```python
from build123d import *

# Parameters (mm, degrees)
BOSS_EXTRU_1_DEPTH                                 = 50
CHAMBRAGE_POUR_VIS_T_TE_HEXAGONALE_M62_D           = 6.6
CHAMBRAGE_POUR_VIS_T_TE_HEXAGONALE_M62_CBORE_D     = 11
CHAMBRAGE_POUR_VIS_T_TE_HEXAGONALE_M62_CBORE_DEPTH = 6.4
ESQUISSE5_R                                        = 10
ENL_V_MAT_EXTRU_1_DEPTH                            = 64.472923802


with BuildPart() as part:
    # Esquisse1 → Boss.-Extru.1 (new body)
    with BuildSketch(Plane.XY):
        with BuildLine():
            Line((-36.108337762, -1), (-36.108337762, -16))
            Line((-36.108337762, -16), (13.891662238, -16))
            Line((13.891662238, -16), (13.891662238, -1))
            Line((13.891662238, -1), (4.898979486, -1))
            ThreePointArc((4.898979486, -1), (0, -5), (-4.898979486, -1))
            Line((-4.898979486, -1), (-36.108337762, -1))
        make_face()
    extrude(amount=BOSS_EXTRU_1_DEPTH)

    # Chambrage pour vis à tête hexagonale M62 (through all)
    with Locations(Plane(origin=(0, -16, 0), x_dir=(-1, 0, 0), z_dir=(0, -1, 0))):
        with Locations((12.108337762, -42), (28.108337762, -8)):
            CounterBoreHole(CHAMBRAGE_POUR_VIS_T_TE_HEXAGONALE_M62_D / 2, CHAMBRAGE_POUR_VIS_T_TE_HEXAGONALE_M62_CBORE_D / 2, CHAMBRAGE_POUR_VIS_T_TE_HEXAGONALE_M62_CBORE_DEPTH)

    # Esquisse5 → Enlèv. mat.-Extru.1 (cut, through all)
    with BuildSketch(Plane(origin=(0, -16, 0), x_dir=(-1, 0, 0), z_dir=(0, -1, 0))):
        with Locations(Location((21.108337762, -25, 0), (0, 0, 90))):
            Circle(ESQUISSE5_R)
    extrude(amount=-ENL_V_MAT_EXTRU_1_DEPTH, mode=Mode.SUBTRACT)


solid = part.part
```
Model file for the job. Use its own axes, mm. A direction names the side the tool comes from. Coordinates: 2 decimals unless noted, no trailing zeros. Loops run counter-clockwise (first coordinate to the right, second up) from the corner with the lowest first, then second, coordinate; pieces in that order, holes last. Notation, with made-up numbers: (-26, -7) -> (-6, -7) arc R20 cw to (-6, 4) -> close; hole circle Ø2 at (-28.5, -2). An arc over 180 degrees is marked (long way). Answer as a JSON object with one key per item and string values.
Q1. Cut at C-C (x = -24). List the corners of the cut face in (y, z), and give its area (3 significant figures).
Report:
{"outline": "(-16, 0) -> (-1, 0) -> (-1, 15.43) -> (-16, 15.43) -> (-16, 11.66) -> (-9.6, 11.66) -> (-9.6, 4.34) -> (-16, 4.34) -> close; (-16, 34.57) -> (-1, 34.57) -> (-1, 50) -> (-16, 50) -> close", "area": "416 mm2"}
Q2. Probe probe 1 along X at (y, z) = (-9, 8); probe 2 along Z at (x, y) = (-15, -13.75); probe 3 along X at (y, z) = (-8.5, 42). List the from-to ranges inside material, lowest first.
Report:
{"probe 1": "x = -36.11 to -31.41, -24.81 to 13.89", "probe 2": "z = 0 to 17.08, 32.92 to 37.32, 46.68 to 50", "probe 3": "x = -36.11 to -15.41, -8.81 to 13.89"}
Q3. Cut at D-D (y = -11.75). List the corners of the cut face in (x, z), and give its area (3 significant figures).
Report:
{"outline": "(-36.11, 0) -> (13.89, 0) -> (13.89, 50) -> (-36.11, 50) -> close; hole circle Ø11 at (-28.11, 8); hole circle Ø20 at (-21.11, 25); hole circle Ø11 at (-12.11, 42)", "area": "2,000 mm2"}
Q4. Cut at B-B (z = 42). List the corners of the cut face in (x, y).
Report:
{"outline": "(-36.11, -16) -> (-17.61, -16) -> (-17.61, -9.6) -> (-15.41, -9.6) -> (-15.41, -1) -> (-36.11, -1) -> close; (-8.81, -9.6) -> (-6.61, -9.6) -> (-6.61, -16) -> (13.89, -16) -> (13.89, -1) -> (4.9, -1) arc R5 cw to (-4.9, -1) -> (-8.81, -1) -> close"}
Q5. Pull direction X, two halves, no side cores. Call faces 3 (the flat face through (-11, -8, 50)), 4 (the flat face through (13.892, -9, 25)), 5 (the cylindrical face through (-11.392, -12.845, 36.547)): released by +X, released by -X, zero draft, split by the parting line, or undercut.
Report:
{"face 3": "zero draft", "face 4": "released by +X", "face 5": "undercut"}
Q6. Cut at A-A (y = -3.5). List the corners of the cut face in (x, z).
Report:
{"outline": "(-36.11, 0) -> (-3.57, 0) -> (-3.57, 50) -> (-36.11, 50) -> close; (3.57, 0) -> (13.89, 0) -> (13.89, 50) -> (3.57, 50) -> close; hole circle Ø6.6 at (-28.11, 8); hole circle Ø20 at (-21.11, 25); hole circle Ø6.6 at (-12.11, 42)"}
Q7. 3-axis set-ups, long thin cutter, end or side, ignore diameter. For faces 1 (the flat face through (-32, -9.6, 8)), 2 (the cylindrical face through (-12.54, -5.24, 38.73)): which of +Z, -Z, +X, -X, +Y, -Y reach the whole face in a straight line?
Report:
{"face 1": "-Y", "face 2": "+Y, -Y"}
Q8. Flat gauge pins, fed straight in: P1, Ø5.5, axis at x = -12, z = 44.5, coming from the -Y side; P2, Ø5.5, axis at x = -28.11, z = 8, coming from the +Y side. Where does each tip first touch, or does it go through?
Report:
{"P1": "stops at y = -9.6", "P2": "passes through"}
